Check sheet for the modelled part. Datum: model origin and axes. Units: mm. A direction names the side the tool comes from. Give positions to 0.01 mm unless a question says otherwise; leave off trailing zeros. Order: outer loops, then holes, each group sorted by start corner. A loop starts at its lowest first (then second) coordinate and runs counter-clockwise, first axis right, second up. Notation, with made-up numbers: (36, 86) - (59, 86) arc R30 cw to (59, 111) - close; hole circle Ø8 at (74, -15). An arc over 180 degrees is marked (long way). Answer in a Markdown table with one row per item.
from build123d import *

# Parameters (mm, degrees)
F0_W     = 5.3
F0_H     = 4
F1_DEPTH = 30
F2_R     = 1.75
F2_R_2   = 1.3
F3_DEPTH = 15
F4_R     = 1.3
F5_DEPTH = 25.8
F6_R     = 2.05
F7_DEPTH = 5
F8_SIZE  = 0.25


with BuildPart() as f1:
    # F0 (on Front) → F1 (new body)
    with BuildSketch(Plane.XZ):
        Rectangle(F0_W, F0_H)
    extrude(amount=-F1_DEPTH)

    # F2 (on face) → F3 (join)
    with BuildSketch(Plane.XZ):
        Circle(F2_R)
        Circle(F2_R_2, mode=Mode.SUBTRACT)
    extrude(amount=F3_DEPTH)

    # F4 (on face) → F5 (join)
    with BuildSketch(Plane.XZ):
        Circle(F4_R)
    extrude(amount=-F5_DEPTH)

    # F6 (on face) → F7 (cut)
    with BuildSketch(Plane(origin=(0, 0, -2), x_dir=(1, 0, 0), z_dir=(0, 0, -1))):
        with Locations((0, -27.128747)):
            Circle(F6_R)
    extrude(amount=-F7_DEPTH, mode=Mode.SUBTRACT)

    # F8
    f8_edges = [f1.edges().sort_by_distance(p)[0] for p in [
        (-2.05, 27.128747, -2),
        (-2.05, 27.128747, 2),
    ]]
    chamfer(f8_edges, length=F8_SIZE)


solid = f1.part
(1) Mould release check, pull along Z, two halves, no side actions. Record for faces 1 (the cylindrical face through (1.617, -7.395, -0.67)), 2 (the flat face through (0, 15, -2)), 3 (the cylindrical face through (-0.17, -7.4, 1.29)): pulls with the +Z half, pulls with the -Z half, needs draft (parallel to the pull), parting line crosses it, or undercut.
Geometry says:
| item | result |
|---|---|
| face 1 | parting line crosses it |
| face 2 | pulls with the -Z half |
| face 3 | undercut |
(2) Thickness scan on L1, parallel to Y at x = -0.1, z = -0.7; L2, parallel to Z at x = 0, y = -9; L3, parallel to Y at x = -2.3, z = -1.3. Record the ranges inside material, lowest first.
Geometry says:
| item | result |
|---|---|
| L1 | 0 to 25.08, 29.18 to 30 |
| L2 | -1.75 to -1.3, 1.3 to 1.75 |
| L3 | 0 to 30 |
(3) Cross-section at A-A, the plane x = 0. Record the cut outline in (y, z), then the cut area to 3 significant figures.
Geometry says:
| item | result |
|---|---|
| outline | (-15, -1.75) - (0, -1.75) - (0, -2) - (24.83, -2) - (25.08, -1.75) - (25.08, 1.75) - (24.83, 2) - (0, 2) - (0, 1.75) - (-15, 1.75) - (-15, 1.3) - (0, 1.3) - (0, -1.3) - (-15, -1.3) - close; (29.18, -1.75) - (29.43, -2) - (30, -2) - (30, 2) - (29.43, 2) - (29.18, 1.75) - close |
| area | 117 mm² |
(4) Access from +Z, -Z, +X, -X, +Y, -Y to the whole of each face (thin tool, end or side, straight path). Record for faces 4 (the flat face through (0, 15, 2)), 5 (the flat face through (-2, 0, 0)).
Geometry says:
| item | result |
|---|---|
| face 4 | +Z, +X, -X, +Y, -Y |
| face 5 | -Y |
(5) Cross-section at B-B, the plane z = 0. Record the cut outline in (x, y), then the cut area to 3 significant figures.
Geometry says:
| item | result |
|---|---|
| outline | (-2.65, 0) - (-1.75, 0) - (-1.75, -15) - (-1.3, -15) - (-1.3, 0) - (1.3, 0) - (1.3, -15) - (1.75, -15) - (1.75, 0) - (2.65, 0) - (2.65, 30) - (-2.65, 30) - close; hole circle Ø4.1 at (0, 27.13) |
| area | 159 mm² |
(6) Gauge pin test, flat ends, axial feed: P1, Ø2, axis at x = 0.5, z = -0.5, coming from the -Y side; P2, Ø1.2, axis at x = 0, z = -0.5, coming from the -Y side. Record the tip position at first contact, or that the pin passes through.
Geometry says:
| item | result |
|---|---|
| P1 | y = -15 |
| P2 | y = 0 |
